from build123d import *

# Parameters (mm, degrees)
F0_W          = 35
F0_H          = 14
F0_R          = 3
F1_DEPTH      = 5
F2_R          = 5.08
F3_R          = 3
F4_DEPTH      = 25.4
F4_DEPTH_BACK = 4.8514


with BuildPart() as f1:
    # F0 (on Front) → F1 (new body)
    with BuildSketch(Plane.XZ):
        with Locations((17.5, 7)):
            Rectangle(F0_W, F0_H)
        with Locations((7, 7)):
            Circle(F0_R, mode=Mode.SUBTRACT)
        with Locations((28, 7)):
            Circle(F0_R, mode=Mode.SUBTRACT)
    extrude(amount=F1_DEPTH)

    # F2
    f2_edges = [f1.edges().sort_by_distance(p)[0] for p in [
        (35, -2.5, 14),
        (35, -2.5, 0),
        (0, -2.5, 0),
        (0, -2.5, 14),
    ]]
    fillet(f2_edges, radius=F2_R)

    # F3 (on face) → F4 (join, two sides)
    with BuildSketch(Plane.XZ.offset(5)) as f4_sk:
        with Locations((28, 7)):
            Circle(F3_R)
        with Locations((7, 7)):
            Circle(F3_R)
    extrude(amount=F4_DEPTH)
    extrude(f4_sk.sketch, amount=-F4_DEPTH_BACK)


solid = f1.part
Can you work these out from the model? Positions are in its coordinate system, mm. A direction names the side the tool comes from. Give positions to 0.01 mm unless a question says otherwise; leave off trailing zeros. Order: outer loops, then holes, each group sorted by start corner. A loop starts at its lowest first (then second) coordinate and runs counter-clockwise, first axis right, second up. Notation, with made-up numbers: M -10,62 L 14,62 A14 ccw 14,73 Z; hole C -26.75,48 d1. An arc over 180 degrees is marked long. Use one line per item in the form item = value.
Item 1: If I drill on line 1 along Y through (x, z) = (24.5, 3.75); line 2 along X through (y, z) = (-2.5, 9); line 3 along Y through (x, z) = (27, 8.5), over which ranges is the centre line in solid material (lowest first)? Write a range as [from, to].
Values follow:
line_1 = [-5, 0]
line_2 = [0, 35]
line_3 = [-30.4, -0.15]
Item 2: If we section it at A-A, the plane x = 7: Write out the boundary of the cut face in (y, z), and give its area (3 significant figures).
Values follow:
outline = M -30.4,4 L -5,4 L -5,0 L 0,0 L 0,4 L -0.15,4 L -0.15,10 L 0,10 L 0,14 L -5,14 L -5,10 L -30.4,10 Z
area = 222 mm^2
Item 3: If we section it at C-C, the plane y = -9.5: Write out the boundary of the cut face in (x, z), and give its area (3 significant figures).
Values follow:
outline = C 7,7 d6; C 28,7 d6
area = 56.5 mm^2
Item 4: Will these pins go through, and if not, where does the flat tip stop? pin 1 Ø4 at (y, z) = (-21, 7.5) entering from +X; pin 2 Ø1 at (y, z) = (-4, 11) entering from -X; pin 3 Ø1 at (y, z) = (-19, 12) entering from -X; pin 4 Ø1.5 at (x, z) = (24, 8) entering from -Y.
Values follow:
pin_1 = 31
pin_2 = 0.25
pin_3 = through
pin_4 = -5
Item 5: If we section it at D-D, the plane x = 24: Write out the boundary of the cut face in (y, z).
Values follow:
outline = M -5,0 L 0,0 L 0,14 L -5,14 Z
Item 6: For faces 1 (the flat face through (28, -0.149, 7)), 2 (the cylindrical face through (25, -18, 7)), 3 (the cylindrical face through (33.472, -2.535, 1.449)), which set-ups out of +Z, -Z, +X, -X, +Y, -Y let a thin tool reach every point of the face, with its end or its side?
Values follow:
face_1 = +Y
face_2 = -Y
face_3 = -Z, +X, +Y, -Y
Item 7: If we section it at B-B, the plane z = 7: Write out the boundary of the cut face in (x, y).
Values follow:
outline = M 0,-5 L 4,-5 L 4,-30.4 L 10,-30.4 L 10,-5 L 25,-5 L 25,-30.4 L 31,-30.4 L 31,-5 L 35,-5 L 35,0 L 31,0 L 31,-0.15 L 25,-0.15 L 25,0 L 10,0 L 10,-0.15 L 4,-0.15 L 4,0 L 0,0 Z
